from build123d import *

# Parameters (mm, degrees)
SKETCH1_W           = 98
SKETCH1_H           = 98
BOSS_EXTRUDE1_DEPTH = 30
SKETCH2_W           = 94
SKETCH2_H           = 94
CUT_EXTRUDE1_DEPTH  = 5
SKETCH3_W           = 90
SKETCH3_H           = 90
CUT_EXTRUDE2_DEPTH  = 21
SKETCH4_W           = 98
SKETCH4_H           = 98
SKETCH4_W_2         = 94
SKETCH4_H_2         = 94
CUT_EXTRUDE3_DEPTH  = 1.8
SKETCH5_R           = 1.3
BOSS_EXTRUDE2_DEPTH = 2.5
FILLET1_R           = 1.5
FILLET2_R           = 1.5
CUT_EXTRUDE4_REACH  = 100
SKETCH6_R           = 8
SKETCH7_R           = 1.968352886
CUT_EXTRUDE5_DEPTH  = 1
SKETCH8_R           = 2.75
BOSS_EXTRUDE3_DEPTH = 3
FILLET3_R           = 5


with BuildPart() as part:
    # Sketch1 → Boss-Extrude1 (new body)
    with BuildSketch(Plane(origin=(0, 0, 0), x_dir=(1, 0, 0), z_dir=(0, 1, 0))):
        Rectangle(SKETCH1_W, SKETCH1_H)
    extrude(amount=BOSS_EXTRUDE1_DEPTH)

    # Sketch2 → Cut-Extrude1 (cut)
    with BuildSketch(Plane(origin=(0, 30, 0), x_dir=(1, 0, 0), z_dir=(0, 1, 0))):
        Rectangle(SKETCH2_W, SKETCH2_H)
    extrude(amount=-CUT_EXTRUDE1_DEPTH, mode=Mode.SUBTRACT)

    # Sketch3 → Cut-Extrude2 (cut)
    with BuildSketch(Plane(origin=(0, 25, 0), x_dir=(1, 0, 0), z_dir=(0, 1, 0))):
        Rectangle(SKETCH3_W, SKETCH3_H)
    extrude(amount=-CUT_EXTRUDE2_DEPTH, mode=Mode.SUBTRACT)

    # Sketch4 → Cut-Extrude3 (cut)
    with BuildSketch(Plane(origin=(0, 30, 0), x_dir=(1, 0, 0), z_dir=(0, 1, 0))):
        Rectangle(SKETCH4_W, SKETCH4_H)
        Rectangle(SKETCH4_W_2, SKETCH4_H_2, mode=Mode.SUBTRACT)
    extrude(amount=-CUT_EXTRUDE3_DEPTH, mode=Mode.SUBTRACT)

    # Sketch5 → Boss-Extrude2 (add)
    with BuildSketch(Plane(origin=(0, 28.2, 0), x_dir=(1, 0, 0), z_dir=(0, 1, 0))):
        with BuildLine():
            Line((-49, 4), (-51, 4))
            ThreePointArc((-51, 4), (-55, 0), (-51, -4))
            Line((-51, -4), (-49, -4))
            Line((-49, -4), (-49, 4))
        make_face()
        with Locations((-52.4, 0)):
            Circle(SKETCH5_R, mode=Mode.SUBTRACT)
        with BuildLine():
            Line((49, 4), (49, -4))
            Line((49, -4), (51, -4))
            ThreePointArc((51, -4), (55, 0), (51, 4))
            Line((51, 4), (49, 4))
        make_face()
        with Locations((52.4, 0)):
            Circle(SKETCH5_R, mode=Mode.SUBTRACT)
    extrude(amount=-BOSS_EXTRUDE2_DEPTH)

    # Fillet1
    fillet1_edges = [part.edges().sort_by_distance(p)[0] for p in [
        (-49, 25.7, 0),
        (-49, 26.95, -4),
        (-49, 26.95, 4),
    ]]
    fillet(fillet1_edges, radius=FILLET1_R)

    # Fillet2
    fillet2_edges = [part.edges().sort_by_distance(p)[0] for p in [
        (49, 26.95, -4),
        (49, 25.7, 0),
        (49, 26.95, 4),
    ]]
    fillet(fillet2_edges, radius=FILLET2_R)

    # Sketch6 → Cut-Extrude4 (cut, up to next)
    with BuildSketch(Plane(origin=(0, 0, -49), x_dir=(-1, 0, 0), z_dir=(0, 0, -1)), mode=Mode.PRIVATE) as cut_extrude4_sk1:
        with Locations((0, 14)):
            Circle(SKETCH6_R)
    cut_extrude4_tool1 = extrude(cut_extrude4_sk1.sketch, amount=-CUT_EXTRUDE4_REACH, mode=Mode.PRIVATE) & part.part
    add(cut_extrude4_tool1.solids().sort_by_distance((0, 14, -49))[0], mode=Mode.SUBTRACT)

    # Sketch7 → Cut-Extrude5 (cut)
    with BuildSketch(Plane.XZ):
        with BuildLine():
            Line((-4, -10), (-1, -10))
            Line((-1, -10), (1, -10))
            ThreePointArc((1, -10), (6, -5), (1, 0))
            ThreePointArc((1, 0), (6, 5), (1, 10))
            Line((1, 10), (-4, 10))
            Line((-4, 10), (-4, -10))
        make_face()
        with Locations((1, 5)):
            Circle(SKETCH7_R, mode=Mode.SUBTRACT)
        with Locations((1, -5)):
            Circle(SKETCH7_R, mode=Mode.SUBTRACT)
    extrude(amount=-CUT_EXTRUDE5_DEPTH, mode=Mode.SUBTRACT)

    # Sketch8 → Boss-Extrude3 (add)
    with BuildSketch(Plane.XY.offset(49)):
        with BuildLine():
            Line((11.648602748, -17), (11.648602748, 0))
            Line((11.648602748, 0), (-12.351397252, 0))
            Line((-12.351397252, 0), (-12.351397252, -17))
            ThreePointArc((-12.351397252, -17), (-0.351397252, -29), (11.648602748, -17))
        make_face()
        with Locations((-0.351397252, -17)):
            Circle(SKETCH8_R, mode=Mode.SUBTRACT)
    extrude(amount=-BOSS_EXTRUDE3_DEPTH)

    # Fillet3
    fillet3_edges = [part.edges().sort_by_distance(p)[0] for p in [
        (-0.351397252, 0, 46),
        (-12.351397252, 0, 47.5),
        (11.648602748, 0, 47.5),
    ]]
    fillet(fillet3_edges, radius=FILLET3_R)


solid = part.part
Geometry: final body of the model. Coordinates: model frame, mm. A direction names the side the tool comes from. Round coordinates to 2 decimals unless told otherwise and drop trailing zeros. Order: outer loops, then holes, each group sorted by start corner. A loop starts at its lowest first (then second) coordinate and runs counter-clockwise, first axis right, second up. Notation, with made-up numbers: (53, -2.5) -> (80, -2.5) arc R21 cw to (80, 21.5) -> close; hole circle Ø6 at (13, 12). An arc over 180 degrees is marked (long way). Put each result on its own line as item: value. Start each with the question number.
Q1. Pull-direction query (Z, two-part tool) for faces 1 (the flat face through (-45.5, 25, -0.2)), 2 (the cylindrical face through (-1, -1, 44)), 3 (the flat face through (-49, 14, 1)); classes: +Z half, -Z half, draft (parallel to the pull), parting line (faces both ways), or undercut.
Q2. Section A-A on z = -30. Return the cut outline in (x, y), and give its area (3 significant figures).
Q3. Reachability of faces 4 (the flat face through (45, 15, 1)), 5 (the cylindrical face through (6, 0.5, -5.1)), 6 (the flat face through (1, 0, -5)) from +Z, -Z, +X, -X, +Y, -Y: full face, straight path, thin tool, end or side. Return the list, or none.
Q4. Line query: probe 1 along X at (y, z) = (10, 43.5); probe 2 along X at (y, z) = (26.55, 0). Output: solid intervals per line, ascending.
Q5. Section B-B on y = 14. Return the cut outline in (x, z).
Q6. First-contact query: pin 1 (6.5 mm diameter, centred on y = 10, z = 13.5, fed in from +X); pin 2 (12 mm diameter, centred on x = 32, z = 26.5, fed in from +Y); pin 3 (6 mm diameter, centred on x = -37, z = -21, fed in from -Y). Flat tips, straight axial feed; report the tip coordinate or a pass-through.
Q7. Section C-C on x = 52.4. Return the cut outline in (y, z).
Q8. Section D-D on x = 9.5. Return the cut outline in (y, z).
Ans:
1. face 1: undercut
1. face 2: -Z half
1. face 3: draft
2. outline: (-49, 0) -> (49, 0) -> (49, 28.2) -> (47, 28.2) -> (47, 25) -> (45, 25) -> (45, 4) -> (-45, 4) -> (-45, 25) -> (-47, 25) -> (-47, 28.2) -> (-49, 28.2) -> close
2. area: 573 mm2
3. face 4: +Y
3. face 5: -Y
3. face 6: -Z, +X, -X, -Y
4. probe 1: x = -49 to -45, 45 to 49
4. probe 2: x = -55 to -53.7, -51.1 to -47, 47 to 51.1, 53.7 to 55
5. outline: (-49, -49) -> (-8, -49) -> (-8, -45) -> (-45, -45) -> (-45, 45) -> (45, 45) -> (45, -45) -> (8, -45) -> (8, -49) -> (49, -49) -> (49, 49) -> (-49, 49) -> close
6. pin 1: stops at x = 49
6. pin 2: stops at y = 4
6. pin 3: stops at y = 0
7. outline: (25.7, -3.75) -> (28.2, -3.75) -> (28.2, -1.3) -> (25.7, -1.3) -> close; (25.7, 1.3) -> (28.2, 1.3) -> (28.2, 3.75) -> (25.7, 3.75) -> close
8. outline: (-23.85, 46) -> (-5, 46) arc R5 cw to (0, 41) -> (0, -49) -> (28.2, -49) -> (28.2, -47) -> (25, -47) -> (25, -45) -> (4, -45) -> (4, 45) -> (25, 45) -> (25, 47) -> (28.2, 47) -> (28.2, 49) -> (-23.85, 49) -> close
